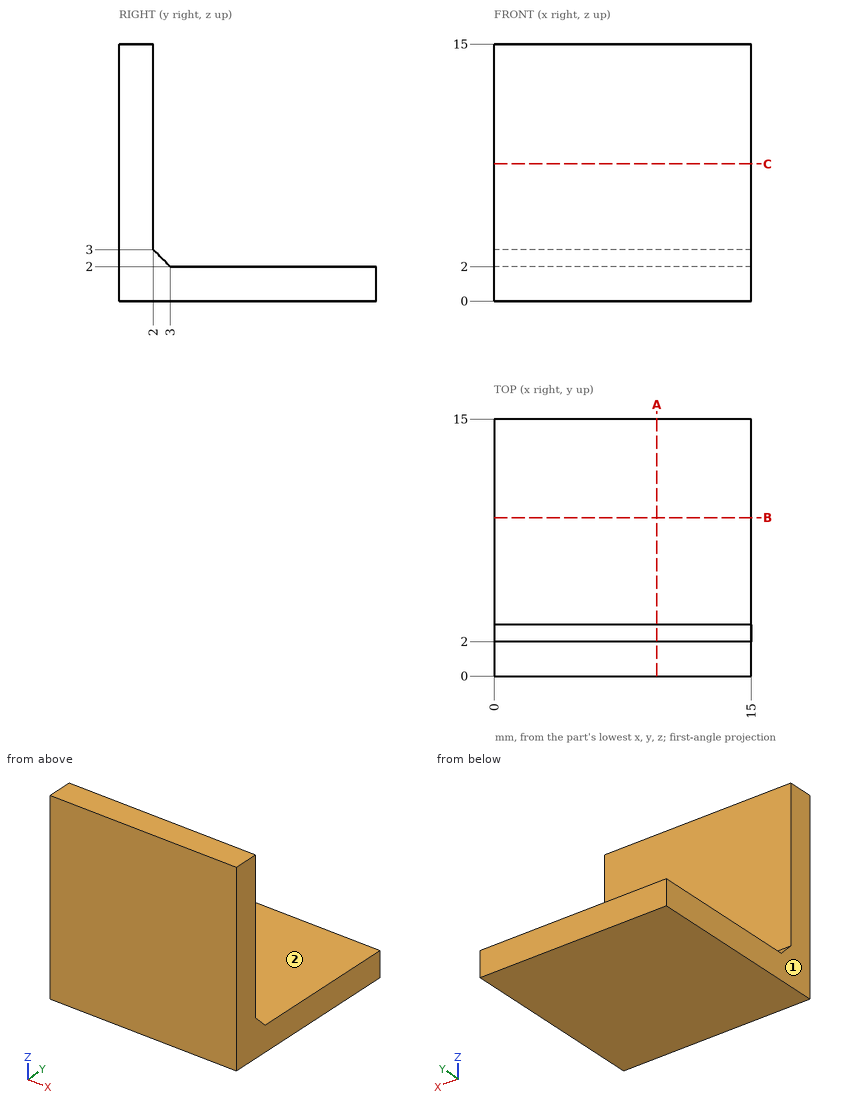
Can you work these out from the drawing? Everything is in mm from the part's minimum corner. A direction names the side the tool comes from. Coordinates: 2 decimals unless noted, no trailing zeros. Write each loop counter-clockwise with the first axis right and the second up, starting at its lowest first coordinate (ties: lowest second). Pieces come first, ordered by that corner, then holes. Notation, with made-up numbers: (5, 69) - (39, 69) arc R11 ccw to (39, 85) - close; hole circle Ø8 at (56.5, 25). An arc over 180 degrees is marked (long way). Use a Markdown table: item, result.
Q1. Please list where these lines run through material, in increasing order: L1, parallel to Z at x = 1.75, y = 10; L2, parallel to Y at x = 8, z = 2.75.
Geometry check:
| item | result |
|---|---|
| L1 | z = 0 to 2 |
| L2 | y = 0 to 2.25 |
Q2. I'm going to push a flat-ended pin straight in: pin 1 Ø5 at (x, z) = (7.5, 13) entering from +Y. Where does the tip first touch, or does it pass through?
Geometry check:
| item | result |
|---|---|
| pin 1 | stops at y = 2 |
Q3. Imagine slicing it at B-B (y = 9.25). List the corners of the cut face in (x, z) for me.
Geometry check:
| item | result |
|---|---|
| outline | (0, 0) - (15, 0) - (15, 2) - (0, 2) - close |
Q4. Imagine slicing it at A-A (x = 9.5). List the corners of the cut face in (y, z) for me.
Geometry check:
| item | result |
|---|---|
| outline | (0, 0) - (15, 0) - (15, 2) - (3, 2) - (2, 3) - (2, 15) - (0, 15) - close |
Q5. Which directions (+Z, -Z, +X, -X, +Y, -Y) give clear straight access to the entire face, cutting with the end or side of a thin tool? Please do the marked faces 1 and 2.
Geometry check:
| item | result |
|---|---|
| face 1 | +Z, -Z, -X, +Y, -Y |
| face 2 | +Z, +X, -X, +Y |
